Input: part model. Units: mm. Frame: model coordinates. A direction names the side the tool comes from. Round coordinates to 2 decimals unless told otherwise and drop trailing zeros. Order: outer loops, then holes, each group sorted by start corner. A loop starts at its lowest first (then second) coordinate and runs counter-clockwise, first axis right, second up. Notation, with made-up numbers: (16, 5) -> (64, 5) arc R17 ccw to (64, 19) -> close; hole circle Ø1 at (77, -22). An arc over 180 degrees is marked (long way). Use a Markdown table: item, result.
from build123d import *

# Parameters (mm, degrees)
SKETCH1_W           = 16
SKETCH1_H           = 30
BOSS_EXTRUDE1_DEPTH = 25
CUT_EXTRUDE1_DEPTH  = 10
SKETCH3_R           = 4.25
CUT_EXTRUDE2_DEPTH  = 34.256578297
FILLET1_R           = 2


with BuildPart() as part:
    # Sketch1 → Boss-Extrude1 (new body)
    with BuildSketch(Plane(origin=(0, 0, 0), x_dir=(1, 0, 0), z_dir=(0, 1, 0))):
        Rectangle(SKETCH1_W, SKETCH1_H)
    extrude(amount=BOSS_EXTRUDE1_DEPTH)

    # Sketch2 → Cut-Extrude1 (cut)
    with BuildSketch(Plane(origin=(0, 25, 0), x_dir=(1, 0, 0), z_dir=(0, 1, 0))):
        with BuildLine():
            Line((-8, 6), (-3.7, 6))
            ThreePointArc((-3.7, 6), (2.3, 0), (-3.7, -6))
            Line((-3.7, -6), (-8, -6))
            ThreePointArc((-8, -6), (-14, 0), (-8, 6))
        make_face()
    extrude(amount=-CUT_EXTRUDE1_DEPTH, mode=Mode.SUBTRACT)

    # Sketch3 → Cut-Extrude2 (cut, through all)
    with BuildSketch(Plane.ZY.offset(8)):
        with Locations((0, 8)):
            Circle(SKETCH3_R)
    extrude(amount=-CUT_EXTRUDE2_DEPTH, mode=Mode.SUBTRACT)

    # Fillet1
    fillet1_edges = [part.edges().sort_by_distance(p)[0] for p in [
        (0, 25, 15),
        (0, 0, 15),
        (0, 0, -15),
        (0, 25, -15),
    ]]
    fillet(fillet1_edges, radius=FILLET1_R)


solid = part.part
1) Cut plane A-A on x = -6. Return loops of the section in (y, z).
Results found:
| item | result |
|---|---|
| outline | (0, -13) arc R2 ccw to (2, -15) -> (23, -15) arc R2 ccw to (25, -13) -> (25, -6) -> (15, -6) -> (15, 6) -> (25, 6) -> (25, 13) arc R2 ccw to (23, 15) -> (2, 15) arc R2 ccw to (0, 13) -> close; hole circle Ø8.5 at (8, 0) |
2) Set-up query: faces 4 (the cylindrical face through (2.3, 20.1, -0.1)), 5 (the cylindrical face through (0.11, 24.4, -14.43)). Return all of +Z, -Z, +X, -X, +Y, -Y with unobstructed straight access to the full face (end or side cutting, diameter ignored); none if empty.
Results found:
| item | result |
|---|---|
| face 4 | -X, +Y |
| face 5 | -Z, +X, -X, +Y |
3) Cut plane D-D on x = 3.5. Return loops of the section in (y, z).
Results found:
| item | result |
|---|---|
| outline | (0, -13) arc R2 ccw to (2, -15) -> (23, -15) arc R2 ccw to (25, -13) -> (25, 13) arc R2 ccw to (23, 15) -> (2, 15) arc R2 ccw to (0, 13) -> close; hole circle Ø8.5 at (8, 0) |
4) Line query: L1, parallel to Y at x = 6.75, z = 0; L2, parallel to Y at x = -3.5, z = 0; L3, parallel to Z at x = 3.25, y = 10.5. Output: solid intervals per line, ascending. Write a range as [from, to].
Results found:
| item | result |
|---|---|
| L1 | y = [0, 3.75], [12.25, 25] |
| L2 | y = [0, 3.75], [12.25, 15] |
| L3 | z = [-15, -3.44], [3.44, 15] |
5) Pin query (flat end, axial travel): pin 1 Ø5 at (x, z) = (-2, -2) entering from +Y. Return the tip coordinate at first contact, or that it passes through.
Results found:
| item | result |
|---|---|
| pin 1 | stops at y = 15 |
6) Cut plane B-B on z = 0. Return loops of the section in (x, y), and give its area (3 significant figures).
Results found:
| item | result |
|---|---|
| outline | (-8, 0) -> (8, 0) -> (8, 3.75) -> (-8, 3.75) -> close; (-8, 12.25) -> (8, 12.25) -> (8, 25) -> (2.3, 25) -> (2.3, 15) -> (-8, 15) -> close |
| area | 161 mm² |
7) Pull-direction query (Z, two-part tool) for faces 1 (the cylindrical face through (0.11, 24.4, 14.43)), 2 (the flat face through (-3, 15, 0)), 3 (the flat face through (-8, 12, 4)); classes: +Z half, -Z half, draft (parallel to the pull), parting line (faces both ways), or undercut.
Results found:
| item | result |
|---|---|
| face 1 | +Z half |
| face 2 | undercut |
| face 3 | draft |
8) Cut plane C-C on y = 8. Return loops of the section in (x, z).
Results found:
| item | result |
|---|---|
| outline | (-8, -15) -> (8, -15) -> (8, -4.25) -> (-8, -4.25) -> close; (-8, 4.25) -> (8, 4.25) -> (8, 15) -> (-8, 15) -> close |
